Work out the finished part from the listing and answer in its coordinate system (mm). A direction names the side the tool comes from. Give positions to 0.01 mm unless a question says otherwise; leave off trailing zeros. Loops run counter-clockwise (first coordinate to the right, second up) from the corner with the lowest first, then second, coordinate; pieces in that order, holes last. Notation, with made-up numbers: (-2.5, 27.5) - (52.5, 27.5) arc R16 ccw to (52.5, 50.5) - close; hole circle Ø9 at (72, 5). An arc over 180 degrees is marked (long way). Use one line per item in the form item = value. Start each with the question number.
from build123d import *

# Parameters (mm, degrees)
BOSS_EXTRUDE1_DEPTH = 152.4
SHELL1_T            = -2.54
SKETCH2_W           = 147.32
SKETCH2_H           = 147.32
CUT_EXTRUDE2_DEPTH  = 152.4


with BuildPart() as part:
    # Sketch1 → Boss-Extrude1 (new body)
    with BuildSketch(Plane(origin=(0, 0, 0), x_dir=(0, 0, -1), z_dir=(1, 0, 0))):
        with BuildLine():
            Line((0, 0), (152.4, 0))
            Line((152.4, 0), (152.4, 25.4))
            ThreePointArc((152.4, 25.4), (159.839487758, 43.360512242), (177.8, 50.8))
            Line((177.8, 50.8), (203.2, 50.8))
            Line((203.2, 50.8), (203.2, 203.2))
            Line((203.2, 203.2), (177.8, 203.2))
            ThreePointArc((177.8, 203.2), (52.076414305, 151.123585695), (0, 25.4))
            Line((0, 25.4), (0, 0))
        make_face()
    extrude(amount=BOSS_EXTRUDE1_DEPTH)

    # Shell1
    shell1_openings = [part.faces().sort_by_distance(p)[0] for p in [
        (76.2, 127, -203.2),
    ]]
    offset(amount=SHELL1_T, openings=shell1_openings, kind=Kind.INTERSECTION)

    # Sketch2 → Cut-Extrude2 (cut)
    with BuildSketch(Plane(origin=(0, 2.54, 0), x_dir=(1, 0, 0), z_dir=(0, 1, 0))):
        with Locations((76.2, 76.2)):
            Rectangle(SKETCH2_W, SKETCH2_H)
    extrude(amount=-CUT_EXTRUDE2_DEPTH, mode=Mode.SUBTRACT)


solid = part.part
1) A cutting plane is placed at B-B (y = 30.5). Give the vertices of the cut face in (x, z).
2) A cutting plane is placed at D-D (y = 77.5). Give the vertices of the cut face in (x, z).
3) A cutting plane is placed at A-A (x = 100.5). Give the vertices of the cut face in (y, z), plus the area to 3 significant figures.
4) A cutting plane is placed at C-C (z = -76.5). Give the vertices of the cut face in (x, y).
5) Determine the mould class of faces 1 (the flat face through (75, 53.34, -190)), 2 (the cylindrical face through (75.13, 152.5, -53.47)), 3 (the cylindrical face through (75.13, 43.16, -159.64)), 4 (the flat face through (42, 53, -203.2)) for opening direction Y: released by +Y, released by -Y, zero draft, split by the parting line, or undercut.
6) Flat-ended cylindrical pins translate along their axes: pin 1 Ø7.5 at (x, z) = (45, -194.5) entering from -Y; pin 2 Ø7.5 at (x, y) = (93, 6.5) entering from -Z; pin 3 Ø1.5 at (x, z) = (132.5, -128.5) entering from -Y. Find the tip coordinate at first contact, or state that the pin passes through.
7) Find the intervals of material crossed by probe 1 along X at (y, z) = (55.5, -137); probe 2 along Z at (x, y) = (82, 9.5); probe 3 along Z at (x, y) = (94, 42.5), in increasing order.
8) A tool of negligible diameter and unlimited length cuts with its end or side. For faces 5 (the flat face through (75, 200.66, -191)), 6 (the flat face through (2.54, 102, -101)), 7 (the flat face through (75, 50.8, -190)), from which of +Z, -Z, +X, -X, +Y, -Y can it reach the whole face along a straight path? Write none if from no direction.
Answer sheet:
q1.outline = (0, -152.92) - (152.4, -152.92) - (152.4, -0.07) - (0, -0.07) - close; hole (2.54, -150.33) - (149.86, -150.33) - (149.86, -2.61) - (2.54, -2.61) - close
q2.outline = (0, -203.2) - (2.54, -203.2) - (2.54, -10.46) - (149.86, -10.46) - (149.86, -203.2) - (152.4, -203.2) - (152.4, -7.8) - (0, -7.8) - close
q3.outline = (0, -152.4) - (25.4, -152.4) arc R25.4 cw to (50.8, -177.8) - (50.8, -203.2) - (53.34, -203.2) - (53.34, -177.8) arc R27.94 ccw to (25.4, -149.86) - (0, -149.86) - close; (0, -2.54) - (25.4, -2.54) arc R175.26 cw to (200.66, -177.8) - (200.66, -203.2) - (203.2, -203.2) - (203.2, -177.8) arc R177.8 ccw to (25.4, 0) - (0, 0) - close
q3.area = 1,070 mm²
q4.outline = (0, 0) - (2.54, 0) - (2.54, 168.42) - (149.86, 168.42) - (149.86, 0) - (152.4, 0) - (152.4, 171.52) - (0, 171.52) - close
q5.face_1 = undercut
q5.face_2 = released by +Y
q5.face_3 = released by -Y
q5.face_4 = zero draft
q6.pin_1 = 50.8
q6.pin_2 = -152.4
q6.pin_3 = 193.36
q7.probe_1 = 0 to 2.54, 149.86 to 152.4
q7.probe_2 = -152.4 to -149.86, -2.54 to 0
q7.probe_3 = -159.02 to -155.7, -3.38 to -0.82
q8.face_5 = -Z
q8.face_6 = none
q8.face_7 = -Z, +X, -X, -Y
